from build123d import *

# Parameters (mm, degrees)
BOSS_EXTRUDE1_DEPTH = 38
SKETCH2_R           = 6.5
CUT_EXTRUDE1_DEPTH  = 58
FILLET1_R           = 1.25


with BuildPart() as part:
    # Sketch1 → Boss-Extrude1 (new body)
    with BuildSketch(Plane.XY):
        with BuildLine():
            Line((-9.5, 0), (9.5, 0))
            Line((9.5, 0), (9.5, 38))
            Line((9.5, 38), (8.25, 38))
            ThreePointArc((8.25, 38), (7.366116524, 37.633883476), (7, 36.75))
            Line((7, 36.75), (7, 2.5))
            Line((7, 2.5), (-7, 2.5))
            Line((-7, 2.5), (-7, 36.75))
            ThreePointArc((-7, 36.75), (-7.366116524, 37.633883476), (-8.25, 38))
            Line((-8.25, 38), (-9.5, 38))
            Line((-9.5, 38), (-9.5, 0))
        make_face()
    extrude(amount=BOSS_EXTRUDE1_DEPTH)

    # Sketch2 → Cut-Extrude1 (cut, through all)
    with BuildSketch(Plane(origin=(9.5, 0, 0), x_dir=(0, 0, -1), z_dir=(1, 0, 0))):
        with Locations((-19, 25)):
            Circle(SKETCH2_R)
    extrude(amount=-CUT_EXTRUDE1_DEPTH, mode=Mode.SUBTRACT)

    # Fillet1
    fillet1_edges = [part.edges().sort_by_distance(p)[0] for p in [
        (-7.366116524, 37.633883476, 0),
        (7.366116524, 37.633883476, 0),
        (7.366116524, 37.633883476, 38),
        (-7.366116524, 37.633883476, 38),
        (-9.5, 0, 19),
        (7, 2.5, 19),
        (-7, 2.5, 19),
        (-7, 19.625, 0),
        (-9.5, 19, 0),
        (0, 0, 0),
        (0, 2.5, 0),
        (7, 19.625, 0),
        (9.5, 19, 0),
        (9.5, 0, 19),
        (0, 0, 38),
        (-9.5, 19, 38),
        (-9.5, 38, 19),
        (9.5, 38, 19),
        (9.5, 19, 38),
        (7, 19.625, 38),
        (-7, 19.625, 38),
        (0, 2.5, 38),
    ]]
    fillet(fillet1_edges, radius=FILLET1_R - 0.0001)  # a hair under: the kernel refuses the full size


solid = part.part
Work out the finished part from the listing and answer in its coordinate system (mm). A direction names the side the tool comes from. Give positions to 0.01 mm unless a question says otherwise; leave off trailing zeros. Use a Markdown table: item, result. Add a question column.
1) Each of these flat-tipped pins is pushed along its axis until it touches: P1, Ø9, axis at x = 0, z = 23, coming from the +Y side; P2, Ø8, axis at x = -7, y = 7, coming from the -Z side. Where does it stop, or does it pass through?
2) The part is cut by section A-A, the plane y = 25. Count the separate pieces of the cut face and the enclosed holes in it, plus the area to 3 significant figures.
3) For a pull along X with two mould halves and no side action, classify faces 6 (the cylindrical face through (0.116, 0.356, 37.624)), 7 (the cylindrical face through (7.376, 37.644, 18.751)), 8 (the cylindrical face through (9.144, 19.249, 37.624)), 9 (the cylindrical face through (-9.144, 37.624, 19.249)) as +X half, -X half, draft (parallel to the pull), parting line (faces both ways), or undercut.
4) Consider line 1 along Y through (x, z) = (8.4, 19); line 2 along X through (y, z) = (5, 2.5); line 3 along Y through (x, z) = (3.5, 4). Determine where each line is inside the solid, lowest interval first.
5) Which of the six approach directions +Z, -Z, +X, -X, +Y, -Y give full straight-line access (tool end or side, diameter ignored) to faces 1 (the cylindrical face through (7.376, 20.019, 0.356)), 2 (the flat face through (0, 2.5, 19)), 3 (the flat face through (-9.5, 15, 19)), 4 (the cylindrical face through (-9.144, 18.751, 37.624)), 5 (the cylindrical face through (7.376, 20.019, 37.644))?
Reported:
| question | item | result |
|---|---|---|
| 1 | P1 | stops at y = 2.5 |
| 1 | P2 | stops at z = 0 |
| 2 | separate pieces | 4 |
| 2 | enclosed holes | 0 |
| 2 | area | 122 mm^2 |
| 3 | face 6 | draft |
| 3 | face 7 | undercut |
| 3 | face 8 | +X half |
| 3 | face 9 | -X half |
| 4 | line 1 | y = 0.01 to 18.5, 31.5 to 37.99 |
| 4 | line 2 | x = -9.5 to -7, 7 to 9.5 |
| 4 | line 3 | y = 0 to 2.5 |
| 5 | face 1 | -Z, +Y |
| 5 | face 2 | +Z, -Z, +Y |
| 5 | face 3 | +Z, -Z, -X, +Y, -Y |
| 5 | face 4 | +Z, -X, +Y, -Y |
| 5 | face 5 | +Z, +Y |
